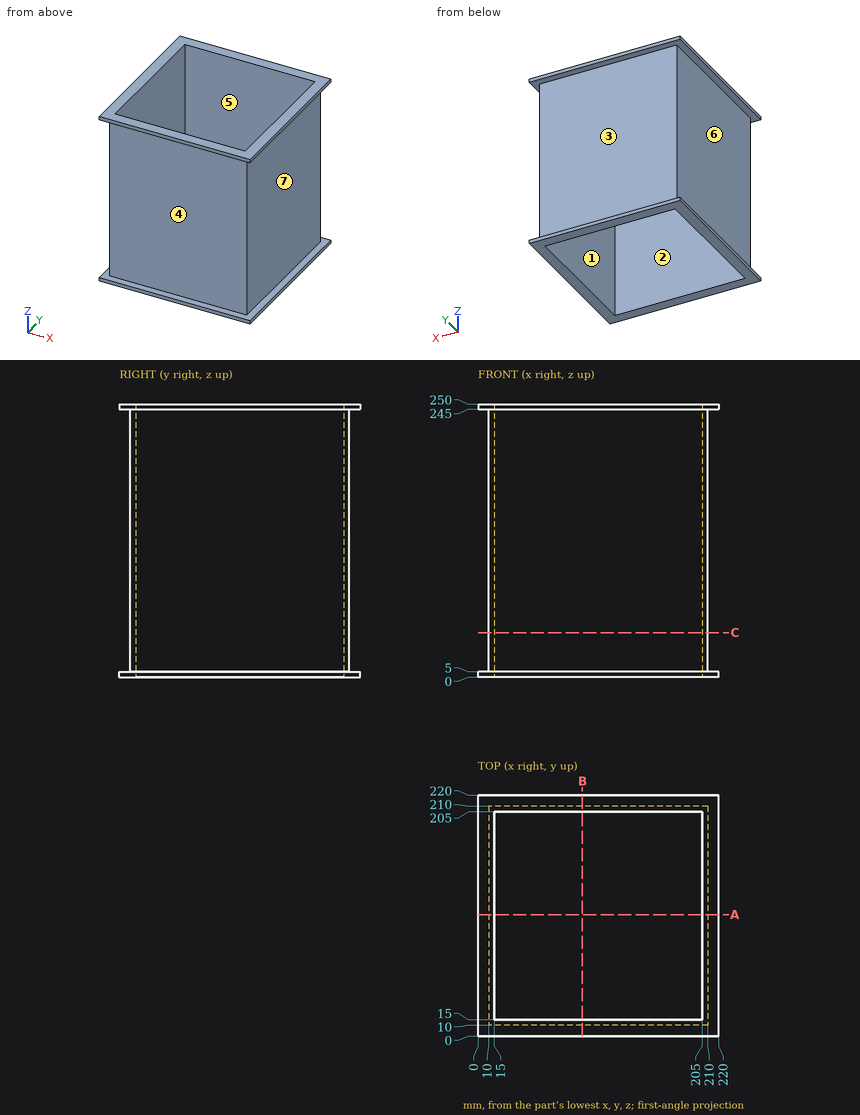
Answer from the drawing. Dimensions are ordinates in mm from the lowest x, y and z of the part. A direction names the side the tool comes from. Coordinates: 2 decimals unless noted, no trailing zeros. Loops run counter-clockwise (first coordinate to the right, second up) from the corner with the lowest first, then second, coordinate; pieces in that order, holes last. Notation, with made-up numbers: (69, -40) -> (107, -40) arc R20 cw to (107, -24) -> close; hole circle Ø5 at (89.25, 28.25). An arc over 180 degrees is marked (long way). Return JSON: item names as keys, results as strings.
Item 1: Find the intervals of material crossed by probe 1 along X at (y, z) = (17.5, 110); probe 2 along X at (y, z) = (209, 83), in increasing order.
Answers:
{"probe 1": "x = 10 to 15, 205 to 210", "probe 2": "x = 10 to 210"}
Item 2: Find section A-A (y = 111). Determine the outline of the cut face in (x, z), plus the area to 3 significant figures.
Answers:
{"outline": "(0, 0) -> (15, 0) -> (15, 250) -> (0, 250) -> (0, 245) -> (10, 245) -> (10, 5) -> (0, 5) -> close; (205, 0) -> (220, 0) -> (220, 5) -> (210, 5) -> (210, 245) -> (220, 245) -> (220, 250) -> (205, 250) -> close", "area": "2,700 mm2"}
Item 3: For a pull along Y with two mould halves and no side action, classify the marked faces 1, 2, 3 and 4 as +Y half, -Y half, draft (parallel to the pull), parting line (faces both ways), or undercut.
Answers:
{"face 1": "undercut", "face 2": "undercut", "face 3": "+Y half", "face 4": "-Y half"}
Item 4: Flat-ended cylindrical pins translate along their axes: P1, Ø8, axis at x = 191, z = 28, coming from the -Y side; P2, Ø5, axis at x = 63, z = 198, coming from the +Y side. Find the tip coordinate at first contact, or state that the pin passes through.
Answers:
{"P1": "stops at y = 10", "P2": "stops at y = 210"}
Item 5: Find section C-C (z = 41). Determine the outline of the cut face in (x, y), plus the area to 3 significant figures.
Answers:
{"outline": "(10, 10) -> (210, 10) -> (210, 210) -> (10, 210) -> close; hole (15, 15) -> (205, 15) -> (205, 205) -> (15, 205) -> close", "area": "3,900 mm2"}
Item 6: For the marked faces 5, 6 and 7, determine the directions among +Z, -Z, +X, -X, +Y, -Y from which every point of the face is accessible in a straight line to the end or side of a thin tool.
Answers:
{"face 5": "+Z, -Z", "face 6": "-X, +Y, -Y", "face 7": "+X, +Y, -Y"}
